Source: CAD feature listing. Evaluate the final solid. Frame: model axes, mm. Face numbers are marked on the shaded views. A direction names the side the tool comes from. Round coordinates to 2 decimals unless told otherwise and drop trailing zeros. Loops run counter-clockwise (first coordinate to the right, second up) from the corner with the lowest first, then second, coordinate; pieces in that order, holes last. Notation, with made-up numbers: M 12,-39 L 32,-39 A33 ccw 32,0 Z; hole C 67,9 d2. An arc over 180 degrees is marked long. Write each question's results on one line, items separated by ' | '. Start each with the question number.
1. Section B-B on y = 0.5. Output: boundary loops of the cut face in (x, z), and give its area (3 significant figures).
2. Section C-C on x = -7.25. Output: boundary loops of the cut face in (y, z).
3. Section D-D on y = -13. Output: boundary loops of the cut face in (x, z).
4. Section A-A on z = 0. Output: boundary loops of the cut face in (x, y), and give its area (3 significant figures).
5. Set-up query: the marked faces 4, 5, 6 and 7. Return all of +Z, -Z, +X, -X, +Y, -Y with unobstructed straight access to the full face (end or side cutting, diameter ignored); none if empty.
6. Draft query along Y for the marked faces 1, 2 and 3. Return one class per face: released by +Y, released by -Y, zero draft, split by the parting line, or undercut.
7. Contact query for flat-ended pins moving along their axis: pin 1 Ø1 at (x, z) = (-10.5, 6) entering from +Y; pin 2 Ø2 at (x, y) = (2.5, 3.5) entering from -Z. Output: stop coordinate, or through.
8. Ray query, line 1 (Y direction, x = 2.25, z = 0); line 2 (X direction, y = -4, z = -7.5); line 3 (Y direction, x = -1, z = 0). Return the intervals inside material, ascending.
from build123d import *

# Parameters (mm, degrees)
BASPROSKE_W      = 10
BASPROSKE_H      = 17
TOOTHCUT_DEPTH   = 27.038433133
TEETHCUTS_COUNT  = 15
TEETHCUTS_ANGLE  = 336
HUBNEAONESKE_R   = 7.5
HUBNEARONE_DEPTH = 13.0000508
BORSKE_R         = 2.5
BORE_DEPTH       = 23.0000508


with BuildPart() as part:
    # BasProSke → Base-Revolve (revolve)
    with BuildSketch(Plane(origin=(0, 0, 0), x_dir=(1, 0, 0), z_dir=(0, 1, 0)), mode=Mode.PRIVATE) as base_revolve_sk:
        with Locations((5, 8.5)):
            Rectangle(BASPROSKE_W, BASPROSKE_H)
    revolve(base_revolve_sk.sketch.rotate(Axis((-10, 0, 0), (1, 0, 0)), 180), axis=Axis((-10, 0, 0), (1, 0, 0)))

    # TooCutSke → ToothCut (cut, through all)
    with BuildSketch(Plane(origin=(0, 0, 0), x_dir=(0, 0, -1), z_dir=(1, 0, 0))):
        with BuildLine():
            ThreePointArc((1.050056448, 12.454813626), (0, 12.499), (-1.050056448, 12.454813626))
            ThreePointArc((-1.050056448, 12.454813626), (-1.638118106, 14.809604533), (-3.110934279, 16.73876737))
            ThreePointArc((-3.110934279, 16.73876737), (0, 17.0254), (3.110934279, 16.73876737))
            ThreePointArc((3.110934279, 16.73876737), (1.638118106, 14.809604533), (1.050056448, 12.454813626))
        make_face()
    toothcut = extrude(amount=TOOTHCUT_DEPTH, mode=Mode.SUBTRACT)

    # TeethCuts: ToothCut ×15 about axis
    teethcuts_axis = Axis((-10, 0, 0), (1, 0, 0))
    for i in range(1, TEETHCUTS_COUNT):
        add(toothcut.rotate(teethcuts_axis, i * TEETHCUTS_ANGLE / (TEETHCUTS_COUNT - 1)), mode=Mode.SUBTRACT)

    # HubNeaOneSke → HubNearOne (add)
    with BuildSketch(Plane.ZY):
        with Locations(Location((0, 0, 0), (0, 0, 180))):
            Circle(HUBNEAONESKE_R)
    extrude(amount=HUBNEARONE_DEPTH)

    # BorSke → Bore (cut, symmetric)
    with BuildSketch(Plane(origin=(0, 0, 0), x_dir=(0, 0, -1), z_dir=(1, 0, 0))):
        with Locations(Location((0, 0, 0), (0, 0, 180))):
            Circle(BORSKE_R)
    extrude(amount=BORE_DEPTH, both=True, mode=Mode.SUBTRACT)


solid = part.part
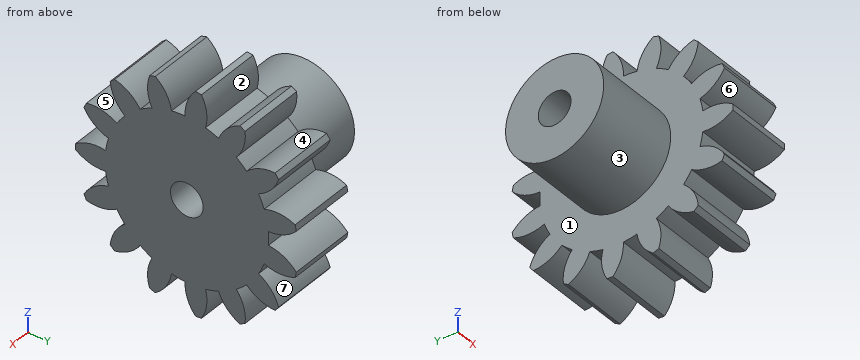
Taken from the geometry:
1) outline: M -13,-7.48 L 0,-7.48 L 0,-15.82 L 10,-15.82 L 10,-2.45 L -13,-2.45 Z; M -13,2.45 L 10,2.45 L 10,15.82 L 0,15.82 L 0,7.48 L -13,7.48 Z | area: 398 mm^2
2) outline: C 0,0 d15; hole C 0,0 d5
3) outline: M 0,-7.39 L 10,-7.39 L 10,-3.99 L 0,-3.99 Z; M 0,-1.63 L 10,-1.63 L 10,1.63 L 0,1.63 Z; M 0,3.99 L 10,3.99 L 10,7.39 L 0,7.39 Z
4) outline: M -13,-7.5 L 0,-7.5 L 0,-17 L 10,-17 L 10,-2.5 L -13,-2.5 Z; M -13,2.5 L 10,2.5 L 10,12.5 L 0,12.5 L 0,7.5 L -13,7.5 Z | area: 375 mm^2
5) face 4: +Z, +X, -X | face 5: +X, -X | face 6: +X, -X, -Y | face 7: +X, -X, +Y
6) face 1: zero draft | face 2: undercut | face 3: split by the parting line
7) pin 1: y = 5.1 | pin 2: z = -16.35
8) line 1: -17 to -2.5, 2.5 to 12.5 | line 2: 0 to 10 | line 3: -7.5 to -2.5, 2.5 to 7.5
